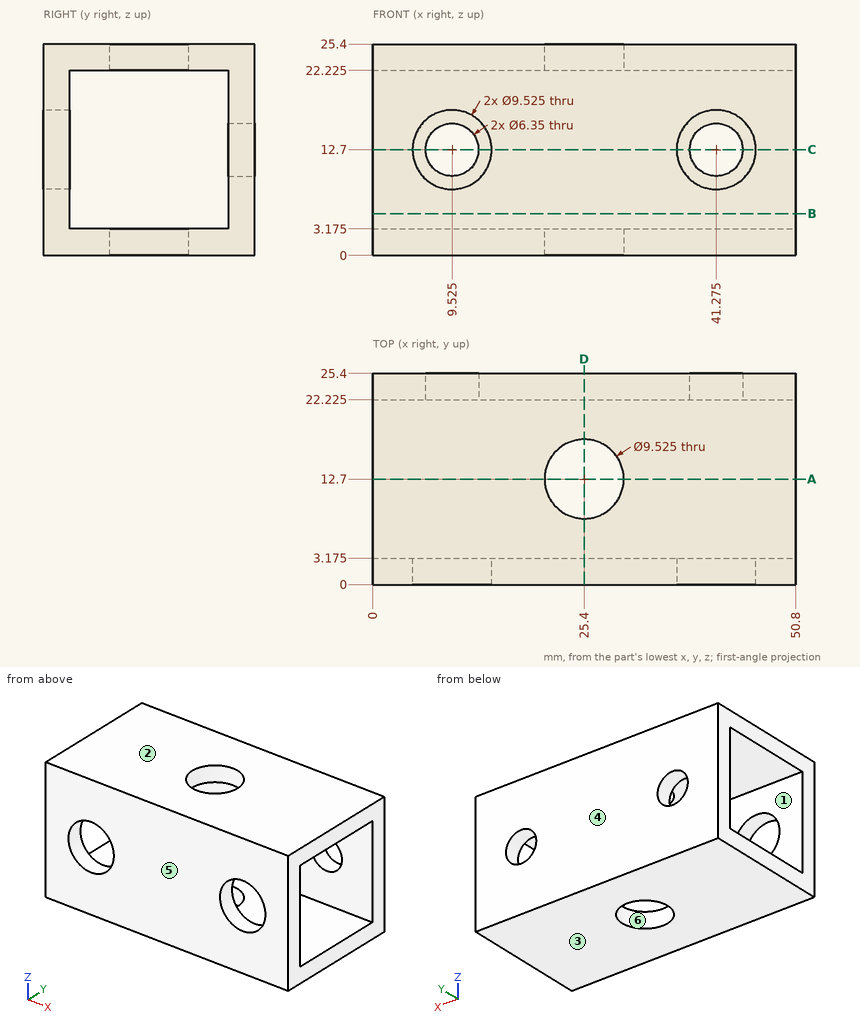
The figure shows three views and two pictorial views of one solid part (mm, origin at its lowest corner). Answer the questions. A direction names the side the tool comes from. Coordinates: 2 decimals unless noted, no trailing zeros. Write each loop counter-clockwise with the first axis right and the second up, starting at its lowest first coordinate (ties: lowest second). Pieces come first, ordered by that corner, then holes. Notation, with made-up numbers: (23.25, 71) -> (33.25, 71) arc R21 cw to (33.25, 109) -> close; hole circle Ø3 at (41.5, 75.25). An arc over 180 degrees is marked (long way). Return JSON: item names as keys, results as strings.
(1) Consider line 1 along Y through (x, z) = (9.5, 18) (3 decimals); line 2 along Y through (x, z) = (25.4, 23.2). Determine where each line is inside the solid, lowest interval first. Write a range as from..to.
Answers below:
{"line 1": "0..3.175, 22.225..25.4", "line 2": "0..7.94, 17.46..25.4"}
(2) Which of the six approach directions +Z, -Z, +X, -X, +Y, -Y give full straight-line access (tool end or side, diameter ignored) to the marked faces 1 and 2?
Answers below:
{"face 1": "+X, -X", "face 2": "+Z, +X, -X, +Y, -Y"}
(3) The part is cut by section D-D on x = 25.4. Give the vertices of the cut face in (y, z) (1 decimal).
Answers below:
{"outline": "(0, 0) -> (7.9, 0) -> (7.9, 3.2) -> (3.2, 3.2) -> (3.2, 22.2) -> (7.9, 22.2) -> (7.9, 25.4) -> (0, 25.4) -> close; (17.5, 0) -> (25.4, 0) -> (25.4, 25.4) -> (17.5, 25.4) -> (17.5, 22.2) -> (22.2, 22.2) -> (22.2, 3.2) -> (17.5, 3.2) -> close"}
(4) The part is cut by section A-A on y = 12.7. Give the vertices of the cut face in (x, z) (1 decimal).
Answers below:
{"outline": "(0, 0) -> (20.6, 0) -> (20.6, 3.2) -> (0, 3.2) -> close; (0, 22.2) -> (20.6, 22.2) -> (20.6, 25.4) -> (0, 25.4) -> close; (30.2, 0) -> (50.8, 0) -> (50.8, 3.2) -> (30.2, 3.2) -> close; (30.2, 22.2) -> (50.8, 22.2) -> (50.8, 25.4) -> (30.2, 25.4) -> close"}
(5) For a pull along Y with two mould halves and no side action, classify the marked faces 3, 4, 5 and 6 as pulls with the +Y half, pulls with the -Y half, needs draft (parallel to the pull), parting line crosses it, or undercut.
Answers below:
{"face 3": "needs draft", "face 4": "pulls with the +Y half", "face 5": "pulls with the -Y half", "face 6": "undercut"}
(6) The part is cut by section C-C on z = 12.7. State how many separate pieces and enclosed holes the cut face has, then the cut area to 3 significant figures.
Answers below:
{"separate pieces": "6", "enclosed holes": "0", "area": "222 mm^2"}
(7) The part is cut by section B-B on z = 5. Give the vertices of the cut face in (x, y) (3 decimals).
Answers below:
{"outline": "(0, 0) -> (50.8, 0) -> (50.8, 3.175) -> (0, 3.175) -> close; (0, 22.225) -> (50.8, 22.225) -> (50.8, 25.4) -> (0, 25.4) -> close"}
(8) This flat-tipped pin is pushed along its axis until it touches: P1, Ø5.5, axis at x = 41.275, z = 12.7, coming from the +Y side. Where does it stop, or does it pass through?
Answers below:
{"P1": "through"}
